```python
from build123d import *

# Parameters (mm, degrees)
F1_DEPTH = 30
F2_R     = 6
F2_R_2   = 3.2
F3_DEPTH = 7
F4_DEPTH = 25
F5_R     = 6
F6_R     = 1


with BuildPart() as f1:
    # F0 (on Top) → F1 (new body)
    with BuildSketch(Plane.XY):
        with BuildLine():
            Line((14, 0), (9, 0))
            Line((9, 0), (9, -0.6))
            Line((9, -0.6), (0.4699246226, -0.6))
            ThreePointArc((0.4699246226, -0.6), (-5.5, -6), (-11.4699246226, -0.6))
            Line((-11.4699246226, -0.6), (-14, -0.6))
            Line((-14, -0.6), (-14, -13.5))
            Line((-14, -13.5), (14, -13.5))
            Line((14, -13.5), (14, 0))
        make_face()
    extrude(amount=F1_DEPTH)

    # F2 (on face) → F3 (cut)
    with BuildSketch(Plane.XZ.offset(13.5)):
        with Locations((4.8, 15)):
            Circle(F2_R)
        with Locations((4.8, 15)):
            Circle(F2_R_2, mode=Mode.SUBTRACT)
    extrude(amount=-F3_DEPTH, mode=Mode.SUBTRACT)

    # F4 (cut): a face of the model
    f4_faces = [f1.faces().sort_by_distance(p)[0] for p in [
        (4.8, -13.5, 15),
    ]]
    extrude(f4_faces, amount=-F4_DEPTH, mode=Mode.SUBTRACT)

    # F5
    f5_edges = [f1.edges().sort_by_distance(p)[0] for p in [
        (14, -6.75, 0),
        (14, -6.75, 30),
    ]]
    fillet(f5_edges, radius=F5_R)

    # F6
    f6_edges = [f1.edges().sort_by_distance(p)[0] for p in [
        (-3, -13.5, 30),
        (-14, -13.5, 15),
        (-14, -7.05, 30),
        (-14, -7.05, 0),
        (-1.2, -13.5, 15),
    ]]
    fillet(f6_edges, radius=F6_R)


solid = f1.part
```
Geometry: final body of the model. Coordinates: model frame, mm. A direction names the side the tool comes from. Give positions to 0.01 mm unless a question says otherwise; leave off trailing zeros. Loops run counter-clockwise (first coordinate to the right, second up) from the corner with the lowest first, then second, coordinate; pieces in that order, holes last. Notation, with made-up numbers: (-15, 89) -> (33, 89) arc R19 cw to (33, 97) -> close; hole circle Ø6 at (68, 12.25). An arc over 180 degrees is marked (long way). Use one line per item in the form item = value.
Item 1: Draft query along X for faces 4 (the face through (-13.699, -13.215, 15.196)), 5 (the face through (7, -6.5, 12)), 6 (the face through (-5.4, -6, 14.8)), 7 (the face through (12.289, -6.162, 28.196)). Return one class per face: pulls with the +X half, pulls with the -X half, needs draft (parallel to the pull), parting line crosses it, or undercut.
A:
face_4 = pulls with the -X half
face_5 = undercut
face_6 = undercut
face_7 = pulls with the +X half
Item 2: Section query C-C on z = 15. Output: boundary loops of the cut face in (x, y).
A:
outline = (-14, -12.5) arc R1 ccw to (-13, -13.5) -> (-2.2, -13.5) arc R1 ccw to (-1.2, -12.5) -> (-1.2, -6.5) -> (1.6, -6.5) -> (1.6, -0.6) -> (0.47, -0.6) arc R6 cw to (-11.47, -0.6) -> (-14, -0.6) -> close; (8, -6.5) -> (10.8, -6.5) -> (10.8, -12.5) arc R1 ccw to (11.8, -13.5) -> (13, -13.5) arc R1 ccw to (14, -12.5) -> (14, 0) -> (9, 0) -> (9, -0.6) -> (8, -0.6) -> close
Item 3: Section query B-B on x = 4.8. Output: boundary loops of the cut face in (y, z).
A:
outline = (-13.5, 1) arc R1 ccw to (-12.5, 0) -> (-0.6, 0) -> (-0.6, 11.8) -> (-6.5, 11.8) -> (-6.5, 9) -> (-12.5, 9) arc R1 ccw to (-13.5, 8) -> close; (-13.5, 22) arc R1 ccw to (-12.5, 21) -> (-6.5, 21) -> (-6.5, 18.2) -> (-0.6, 18.2) -> (-0.6, 30) -> (-12.5, 30) arc R1 ccw to (-13.5, 29) -> close
Item 4: Section query A-A on y = -1.5. Output: boundary loops of the cut face in (x, z), and give its area (3 significant figures).
A:
outline = (-14, 1) arc R1 ccw to (-13, 0) -> (-11.31, 0) -> (-11.31, 30) -> (-13, 30) arc R1 ccw to (-14, 29) -> close; (0.31, 0) -> (8, 0) arc R6 ccw to (14, 6) -> (14, 24) arc R6 ccw to (8, 30) -> (0.31, 30) -> close; hole circle Ø6.4 at (4.8, 15)
area = 443 mm^2
Item 5: Line query: probe 1 along Z at (x, y) = (4.8, -9.05); probe 2 along Z at (x, y) = (4.8, -3.35); probe 3 along Y at (x, z) = (4.75, 24). Output: solid intervals per line, ascending.
A:
probe_1 = 0 to 9, 21 to 30
probe_2 = 0 to 11.8, 18.2 to 30
probe_3 = -13.5 to -0.6
Item 6: Section query D-D on y = -10.75. Output: boundary loops of the cut face in (x, z).
A:
outline = (-14, 1) arc R1 ccw to (-13, 0) -> (8, 0) arc R6 ccw to (14, 6) -> (14, 24) arc R6 ccw to (8, 30) -> (-13, 30) arc R1 ccw to (-14, 29) -> close; hole circle Ø12 at (4.8, 15)
Item 7: Access query for faces 1 (the face through (14, -6, 15)), 2 (the face through (5, -0.6, 11)), 3 (the face through (10.523, -9.542, 16.802)). Directions: +Z, -Z, +X, -X, +Y, -Y. A direction counts if a zero-diameter tool reaches every point of the face in a straight line with its end or side. Return the directions, or none.
A:
face_1 = +Z, -Z, +X, +Y, -Y
face_2 = +Z, -Z, -X, +Y
face_3 = -Y
Item 8: Pin query (flat end, axial travel): P1, Ø1.3, axis at x = -13.5, z = 18, coming from the +Y side; P2, Ø10, axis at x = 4.8, z = 15, coming from the +Y side; P3, Ø1, axis at x = -4.5, z = 19.5, coming from the +Y side. Return the tip coordinate at first contact, or that it passes through.
A:
P1 = -0.6
P2 = 0
P3 = -5.81
